from build123d import *

# Parameters (mm, degrees)
F0_W        = 2.5
F0_H        = 3.8657399043
F1_DEPTH    = 25
F2_T1_DEPTH = 25
F2_T3_DEPTH = 25
F2_T5_DEPTH = 50
F2_T7_DEPTH = 50
F3_T1_DEPTH = 49.8746859277


# Not quite as in the source:
# - a fillet or chamfer that OpenCascade refuses, or shapes differently, is made with other operations: its cross-section is extruded or revolved along the edge and cut away or added


with BuildPart() as f1:
    # F0 (on Right) → F1 (new body)
    with BuildSketch(Plane.YZ):
        Polygon((4.5518016368, 4.6355622155), (0.0518016368, 4.6355622155), (0.0518016368, -8.8644377845), (4.5518016368, -8.8644377845), (4.5518016368, -4.8644377845), (9.0518016368, -4.8644377845), (9.0518016368, -15.2773326263), (11.5518016368, -15.2773326263), (11.5518016368, -11.7773326263), (11.5518016368, 15.966644237), (9.0518016368, 15.966644237), (9.0518016368, -1.3644377845), (4.5518016368, -1.3644377845), align=None)
        Polygon((11.5518016368, -11.7773326263), (11.5518016368, -15.2773326263), (36.5518016368, -15.2773326263), (36.5518016368, -11.7773326263), (34.0518016368, -11.7773326263), align=None)
        with Locations((35.3018016368, -9.8444626741)):
            Rectangle(F0_W, F0_H)
    extrude(amount=F1_DEPTH)

    # F2: fillet of radius 5 on 4 edges, made by hand

    # F2_s2 → F2_t1 (join)
    with BuildSketch(Plane.YZ):
        with BuildLine():
            ThreePointArc((34.0518016368, -7.9115927219), (32.2909091759, -10.6934084988), (29.1821554448, -11.7773326263))
            Line((29.1821554448, -11.7773326263), (34.0518016368, -11.7773326263))
            Line((34.0518016368, -11.7773326263), (34.0518016368, -7.9115927219))
        make_face()
    extrude(amount=F2_T1_DEPTH)

    # F2_s4 → F2_t3 (join)
    with BuildSketch(Plane.YZ):
        with BuildLine():
            ThreePointArc((16.5518016368, -11.7773326263), (13.0162677309, -10.3128665322), (11.5518016368, -6.7773326263))
            Line((11.5518016368, -6.7773326263), (11.5518016368, -11.7773326263))
            Line((11.5518016368, -11.7773326263), (16.5518016368, -11.7773326263))
        make_face()
    extrude(amount=F2_T3_DEPTH)

    # F2_s6 → F2_t5 (cut)
    with BuildSketch(Plane.YZ.offset(-12.5)):
        with BuildLine():
            ThreePointArc((9.0518016368, -10.2773326263), (10.5162677309, -13.8128665322), (14.0518016368, -15.2773326263))
            Line((14.0518016368, -15.2773326263), (9.0518016368, -15.2773326263))
            Line((9.0518016368, -15.2773326263), (9.0518016368, -10.2773326263))
        make_face()
    extrude(amount=F2_T5_DEPTH, mode=Mode.SUBTRACT)

    # F2_s8 → F2_t7 (cut)
    with BuildSketch(Plane.YZ.offset(-12.5)):
        with BuildLine():
            ThreePointArc((36.5518016368, -10.2773326263), (35.0873355427, -13.8128665322), (31.5518016368, -15.2773326263))
            Line((31.5518016368, -15.2773326263), (36.5518016368, -15.2773326263))
            Line((36.5518016368, -15.2773326263), (36.5518016368, -10.2773326263))
        make_face()
    extrude(amount=F2_T7_DEPTH, mode=Mode.SUBTRACT)

    # F3: fillet of radius 5 on 1 edges, made by hand

    # F3_s2 → F3_t1 (cut)
    with BuildSketch(Plane.YZ.offset(-12.4373429638)):
        with BuildLine():
            ThreePointArc((0.0518016368, -3.889500599), (1.3437023933, -7.2436025653), (4.5518016368, -8.8644377845))
            Line((4.5518016368, -8.8644377845), (0.0518016368, -8.8644377845))
            Line((0.0518016368, -8.8644377845), (0.0518016368, -3.889500599))
        make_face()
    extrude(amount=F3_T1_DEPTH, mode=Mode.SUBTRACT)


solid = f1.part
Design review of the part built by this model. Coordinates are the model's own, in mm. A direction names the side the tool comes from. Coordinates: 2 decimals unless noted, no trailing zeros. Order: outer loops, then holes, each group sorted by start corner. A loop starts at its lowest first (then second) coordinate and runs counter-clockwise, first axis right, second up. Notation, with made-up numbers: (-5, 80) -> (25, 80) arc R23 cw to (25, 103) -> close; hole circle Ø11 at (89, 32). An arc over 180 degrees is marked (long way). Use one line per item in the form item = value. Start each with the question number.
(1) For probe 1 along Y at (x, z) = (3, -1); probe 2 along Z at (x, y) = (7.5, 22); probe 3 along Y at (x, z) = (7, -2.5), list the stretches that pass through material, from the lowest coordinate up.
(2) Add section D-D on y = 32.5. State the section outline as (x, z) points.
(3) Add section C-C on z = 12. State the section outline as (x, y) points.
(4) Add section B-B on x = 19.5. State the section outline as (y, z) points, plus the area to 3 significant figures.
(5) For faces 4 (the flat face through (12, 23, -15.277)), 5 (the flat face through (12, 11.552, 4)), 6 (the flat face through (12, 9.052, -8)), 7 (the cylindrical face through (12.32, 32.33, -10.66)), list the 3-axis set-ups (+Z, -Z, +X, -X, +Y, -Y) from which the entire face can be reached by the end or side of a thin tool; tool diameter is ignored.
(6) Add section A-A on z = 4. State the section outline as (x, y) points, plus the area to 3 significant figures.
(7) The part is to be moulded in two halves that separate along Y. For faces 1 (the flat face through (12, 2, 4.636)), 2 (the flat face through (12, 36.552, -9)), 3 (the flat face through (12, 23, -11.777)), say which applies: +Y half, -Y half, draft (parallel to the pull), parting line (faces both ways), or undercut.
(8) Insertion check: pin 1 (4 mm diameter, centred on x = 13, y = 22, fed in from +Z); pin 2 (5 mm diameter, centred on x = 6.5, z = 10, fed in from -Y); pin 3 (8 mm diameter, centred on x = 2.5, z = -2, fed in from +Y); pin 4 (4.5 mm diameter, centred on x = 17, z = -7, fed in from +Y). Each pin has a flat end and moves straight along its axis. Give the tip position at first contact, or say it passes through.
Answer block:
q1.probe_1 = 0.05 to 4.55, 9.05 to 11.55
q1.probe_2 = -15.28 to -11.78
q1.probe_3 = 0.05 to 11.55
q2.outline = (0, -15.19) -> (25, -15.19) -> (25, -10.52) -> (0, -10.52) -> close
q3.outline = (0, 9.05) -> (25, 9.05) -> (25, 11.55) -> (0, 11.55) -> close
q4.outline = (0.05, -3.89) arc R5 ccw to (4.55, -8.86) -> (4.55, -4.86) -> (9.05, -4.86) -> (9.05, -10.28) arc R5 ccw to (14.05, -15.28) -> (31.55, -15.28) arc R5 ccw to (36.55, -10.28) -> (36.55, -7.91) -> (34.05, -7.91) arc R5 cw to (29.18, -11.78) -> (16.55, -11.78) arc R5 cw to (11.55, -6.78) -> (11.55, 15.97) -> (9.05, 15.97) -> (9.05, -1.36) -> (4.55, -1.36) -> (4.55, 4.64) -> (0.05, 4.64) -> close
q4.area = 246 mm²
q5.face_4 = -Z, +X, -X, +Y, -Y
q5.face_5 = +Z, +X, -X, +Y
q5.face_6 = -Z, +X, -X
q5.face_7 = +Z, +X, -X
q6.outline = (0, 0.05) -> (25, 0.05) -> (25, 4.55) -> (0, 4.55) -> close; (0, 9.05) -> (25, 9.05) -> (25, 11.55) -> (0, 11.55) -> close
q6.area = 175 mm²
q7.face_1 = draft
q7.face_2 = +Y half
q7.face_3 = undercut
q8.pin_1 = -11.78
q8.pin_2 = 9.05
q8.pin_3 = 11.55
q8.pin_4 = 36.55
